Verification items for the finished model (mm, model axes). Face numbers are marked on the shaded views. A direction names the side the tool comes from. Coordinates: 2 decimals unless noted, no trailing zeros. Write each loop counter-clockwise with the first axis right and the second up, starting at its lowest first coordinate (ties: lowest second). Pieces come first, ordered by that corner, then holes.
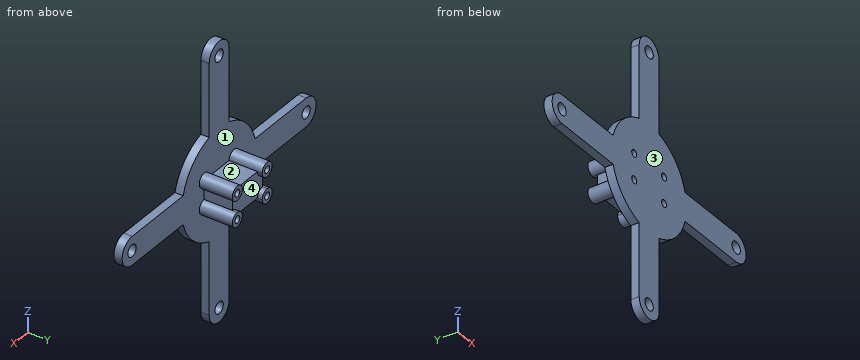
```python
from build123d import *
from build123d.topology import SkipClean

# Parameters (mm, degrees)
SKETCH1_R           = 2.5
BOSS_EXTRUDE1_DEPTH = 3.5
SKETCH4_R           = 1.5
BOSS_EXTRUDE2_DEPTH = 14
CUT_EXTRUDE4_START  = -2
CUT_EXTRUDE4_DEPTH  = 2
CUT_EXTRUDE2_START  = -10
SKETCH4_2_R         = 1.5
CUT_EXTRUDE2_DEPTH  = 10


with BuildPart() as part:
    # Sketch1 → Boss-Extrude1 (new body)
    with BuildSketch(Plane(origin=(0, 0, 0), x_dir=(1, 0, 0), z_dir=(0, 1, 0))):
        with BuildLine():
            Line((-21.685248442, 6), (-52.5, 6))
            ThreePointArc((-52.5, 6), (-58.5, 0), (-52.5, -6))
            Line((-52.5, -6), (-21.685248442, -6))
            ThreePointArc((-21.685248442, -6), (-15.909902577, -15.909902577), (-6, -21.685248442))
            Line((-6, -21.685248442), (-6, -52.5))
            ThreePointArc((-6, -52.5), (0, -58.5), (6, -52.5))
            Line((6, -52.5), (6, -21.685248442))
            ThreePointArc((6, -21.685248442), (15.909902577, -15.909902577), (21.685248442, -6))
            Line((21.685248442, -6), (52.5, -6))
            ThreePointArc((52.5, -6), (58.5, 0), (52.5, 6))
            Line((52.5, 6), (21.685248442, 6))
            ThreePointArc((21.685248442, 6), (15.909902577, 15.909902577), (6, 21.685248442))
            Line((6, 21.685248442), (6, 52.5))
            ThreePointArc((6, 52.5), (0, 58.5), (-6, 52.5))
            Line((-6, 52.5), (-6, 21.685248442))
            ThreePointArc((-6, 21.685248442), (-15.909902577, 15.909902577), (-21.685248442, 6))
        make_face()
        with Locations(Location((0, -52.5, 0), (0, 0, 270))):
            Circle(SKETCH1_R, mode=Mode.SUBTRACT)
        with Locations(Location((52.5, 0, 0), (0, 0, 270))):
            Circle(SKETCH1_R, mode=Mode.SUBTRACT)
        with Locations(Location((-52.5, 0, 0), (0, 0, 270))):
            Circle(SKETCH1_R, mode=Mode.SUBTRACT)
        with Locations(Location((0, 52.5, 0), (0, 0, 270))):
            Circle(SKETCH1_R, mode=Mode.SUBTRACT)
    extrude(amount=BOSS_EXTRUDE1_DEPTH)

    # Sketch4 → Boss-Extrude2 (add)
    with BuildSketch(Plane(origin=(0, 3.5, 0), x_dir=(1, 0, 0), z_dir=(0, 1, 0))):
        with BuildLine():
            Line((-6, -5.5), (6, -5.5))
            ThreePointArc((6, -5.5), (11.121320344, -7.621320344), (9, -2.5))
            Line((9, -2.5), (9, 2.5))
            ThreePointArc((9, 2.5), (11.121320344, 7.621320344), (6, 5.5))
            Line((6, 5.5), (-6, 5.5))
            ThreePointArc((-6, 5.5), (-11.121320344, 7.621320344), (-9, 2.5))
            Line((-9, 2.5), (-9, -2.5))
            ThreePointArc((-9, -2.5), (-11.121320344, -7.621320344), (-6, -5.5))
        make_face()
        with Locations(Location((9, -5.5, 0), (0, 0, 270))):
            Circle(SKETCH4_R, mode=Mode.SUBTRACT)
        with Locations(Location((-9, -5.5, 0), (0, 0, 270))):
            Circle(SKETCH4_R, mode=Mode.SUBTRACT)
        with Locations(Location((-9, 5.5, 0), (0, 0, 270))):
            Circle(SKETCH4_R, mode=Mode.SUBTRACT)
        with Locations(Location((9, 5.5, 0), (0, 0, 270))):
            Circle(SKETCH4_R, mode=Mode.SUBTRACT)
    extrude(amount=BOSS_EXTRUDE2_DEPTH)

    # Sketch6 → Cut-Extrude4 (cut)
    with SkipClean():  # the faces are left unmerged after this step: merging them gives an invalid solid
        with BuildSketch(Plane(origin=(0, 17.5, 0), x_dir=(1, 0, 0), z_dir=(0, 1, 0)).offset(CUT_EXTRUDE4_START)):
            with BuildLine():
                ThreePointArc((9, 2.5), (6.878679656, 3.378679656), (6, 5.5))
                Line((6, 5.5), (-6, 5.5))
                ThreePointArc((-6, 5.5), (-6.878679656, 3.378679656), (-9, 2.5))
                Line((-9, 2.5), (-9, -2.5))
                ThreePointArc((-9, -2.5), (-6.878679656, -3.378679656), (-6, -5.5))
                Line((-6, -5.5), (6, -5.5))
                ThreePointArc((6, -5.5), (6.878679656, -3.378679656), (9, -2.5))
                Line((9, -2.5), (9, 2.5))
            make_face()
        extrude(amount=CUT_EXTRUDE4_DEPTH, mode=Mode.SUBTRACT)

    # Sketch4_2 → Cut-Extrude2 (cut)
    with SkipClean():  # the faces are left unmerged after this step: merging them gives an invalid solid
        with BuildSketch(Plane(origin=(0, 3.5, 0), x_dir=(1, 0, 0), z_dir=(0, 1, 0)).offset(CUT_EXTRUDE2_START)):
            with Locations(Location((-9, -5.5, 0), (0, 0, 270))):
                Circle(SKETCH4_2_R)
            with Locations(Location((9, -5.5, 0), (0, 0, 270))):
                Circle(SKETCH4_2_R)
            with Locations(Location((-9, 5.5, 0), (0, 0, 270))):
                Circle(SKETCH4_2_R)
            with Locations(Location((9, 5.5, 0), (0, 0, 270))):
                Circle(SKETCH4_2_R)
        extrude(amount=CUT_EXTRUDE2_DEPTH, mode=Mode.SUBTRACT)


solid = part.part
```
1. Sectioned sample at A-A, the plane x = 0. Record the boundary of the cut face in (y, z), and give its area (4 significant figures).
2. Material ranges on L1, parallel to X at y = 1.55, z = 0; L2, parallel to Z at x = 9.5, y = 8.25; L3, parallel to Y at x = -23, z = 0, recorded low to high.
3. Sectioned sample at C-C, the plane z = 0. Record the boundary of the cut face in (x, y), and give its area (4 significant figures).
4. Sectioned sample at D-D, the plane x = -26. Record the boundary of the cut face in (y, z).
5. Sectioned sample at B-B, the plane y = 11.25. Record the boundary of the cut face in (x, z).
6. Gauge pin test, flat ends, axial feed: P1, Ø4, axis at x = 29.5, y = 1.5, coming from the -Z side; P2, Ø10, axis at y = 9.5, z = 0.5, coming from the +X side; P3, Ø1, axis at y = 1, z = -43, coming from the +X side; P4, Ø10, axis at x = 17.5, y = 10.5, coming from the -Z side. Record the tip position at first contact, or that the pin passes through.
7. Tool access check on the marked faces 1 and 2. Record the directions out of +Z, -Z, +X, -X, +Y, -Y that give a thin tool (end or side, any length) a straight path to the whole face; none if there is none.
8. Draft check along X on the marked faces 3 and 4. Enter one of: pulls with the +X half, pulls with the -X half, needs draft (parallel to the pull), parting line crosses it, or undercut.
Outcome:
1. outline: (0, -58.5) - (3.5, -58.5) - (3.5, -55) - (0, -55) - close; (0, -50) - (3.5, -50) - (3.5, -5.5) - (15.5, -5.5) - (15.5, 5.5) - (3.5, 5.5) - (3.5, 50) - (0, 50) - close; (0, 55) - (3.5, 55) - (3.5, 58.5) - (0, 58.5) - close
1. area: 506.5 mm2
2. L1: x = -58.5 to -55, -50 to 50, 55 to 58.5
2. L2: z = -8.46 to -6.91, -4.09 to -2.54, 2.54 to 4.09, 6.91 to 8.46
2. L3: y = 0 to 3.5
3. outline: (-58.5, 0) - (-55, 0) - (-55, 3.5) - (-58.5, 3.5) - close; (-50, 0) - (50, 0) - (50, 3.5) - (9, 3.5) - (9, 15.5) - (-9, 15.5) - (-9, 3.5) - (-50, 3.5) - close; (55, 0) - (58.5, 0) - (58.5, 3.5) - (55, 3.5) - close
3. area: 590.5 mm2
4. outline: (0, -6) - (3.5, -6) - (3.5, 6) - (0, 6) - close
5. outline: (-9, -2.5) arc R3 ccw (long way) to (-6, -5.5) - (6, -5.5) arc R3 ccw (long way) to (9, -2.5) - (9, 2.5) arc R3 ccw (long way) to (6, 5.5) - (-6, 5.5) arc R3 ccw (long way) to (-9, 2.5) - close; hole circle Ø3 at (-9, -5.5); hole circle Ø3 at (-9, 5.5); hole circle Ø3 at (9, -5.5); hole circle Ø3 at (9, 5.5)
6. P1: stops at z = -6
6. P2: stops at x = 12
6. P3: stops at x = 6
6. P4: passes through
7. face 1: +Y
7. face 2: +Z, +Y
8. face 3: needs draft
8. face 4: undercut
